Check sheet for the modelled part. Datum: model origin and axes. Units: mm. Face numbers are marked on the shaded views. A direction names the side the tool comes from. Give positions to 0.01 mm unless a question says otherwise; leave off trailing zeros. Write each loop counter-clockwise with the first axis right and the second up, starting at its lowest first coordinate (ties: lowest second). Pieces come first, ordered by that corner, then holes.
from build123d import *

# Parameters (mm, degrees)
SKETCH003_W          = 205
SKETCH003_H          = 151
PAD001_DEPTH         = 40
POCKET002_DEPTH      = 38
SKETCH005_R          = 15
POCKET003_DEPTH      = 2.001
POCKET003_DEPTH_BACK = 38.001
POCKET004_DEPTH      = 38


with BuildPart() as part:
    # Sketch003 → Pad001 (new body)
    with BuildSketch(Plane.XY):
        Rectangle(SKETCH003_W, SKETCH003_H)
    extrude(amount=PAD001_DEPTH)

    # Sketch004 (on Face6 of Pad001) → Pocket002 (cut)
    with BuildSketch(Plane.XY.offset(40)):
        Polygon((-101.5, 0), (-81.2, 35.160631), (-40.6, 35.160631), (-20.3, 70.321263), (20.3, 70.321263), (40.6, 35.160631), (81.2, 35.160631), (101.5, 0), (81.2, -35.160631), (40.6, -35.160631), (19.516262, -71.678737), (-19.516262, -71.678737), (-40.6, -35.160631), (-81.2, -35.160631), align=None)
    extrude(amount=-POCKET002_DEPTH, mode=Mode.SUBTRACT)

    # Sketch005 → Pocket003 (cut, two sides)
    with BuildSketch(Plane.XY.offset(2)) as pocket003_sk:
        with Locations((105, 0)):
            Circle(SKETCH005_R)
        with Locations((0, 75)):
            Circle(SKETCH005_R)
        with Locations((0, -75)):
            Circle(SKETCH005_R)
        with Locations((-105, 0)):
            Circle(SKETCH005_R)
    extrude(amount=-POCKET003_DEPTH, mode=Mode.SUBTRACT)
    extrude(pocket003_sk.sketch, amount=POCKET003_DEPTH_BACK, mode=Mode.SUBTRACT)

    # Sketch006 (on Face6 of Pad001) → Pocket004 (cut)
    with BuildSketch(Plane.XY.offset(40)):
        with BuildLine():
            ThreePointArc((-83.5, -39), (-100.5, -56), (-83.5, -73))
            Line((-83.5, -73), (-50, -73))
            ThreePointArc((-50, -73), (-33, -56), (-50, -39))
            Line((-50, -39), (-83.5, -39))
        make_face()
        with BuildLine():
            ThreePointArc((50, -39), (33, -56), (50, -73))
            Line((50, -73), (83.5, -73))
            ThreePointArc((83.5, -73), (100.5, -56), (83.5, -39))
            Line((83.5, -39), (50, -39))
        make_face()
        with BuildLine():
            ThreePointArc((50, 73), (33, 56), (50, 39))
            Line((50, 39), (83.5, 39))
            ThreePointArc((83.5, 39), (100.5, 56), (83.5, 73))
            Line((83.5, 73), (50, 73))
        make_face()
        with BuildLine():
            ThreePointArc((-83.5, 73), (-100.5, 56), (-83.5, 39))
            Line((-83.5, 39), (-50, 39))
            ThreePointArc((-50, 39), (-33, 56), (-50, 73))
            Line((-50, 73), (-83.5, 73))
        make_face()
    extrude(amount=-POCKET004_DEPTH, mode=Mode.SUBTRACT)


with BuildPart() as part_1:
    # Body001 placement: moved
    add(part.part.moved(Location((100, -60, 0))))


solid = part_1.part
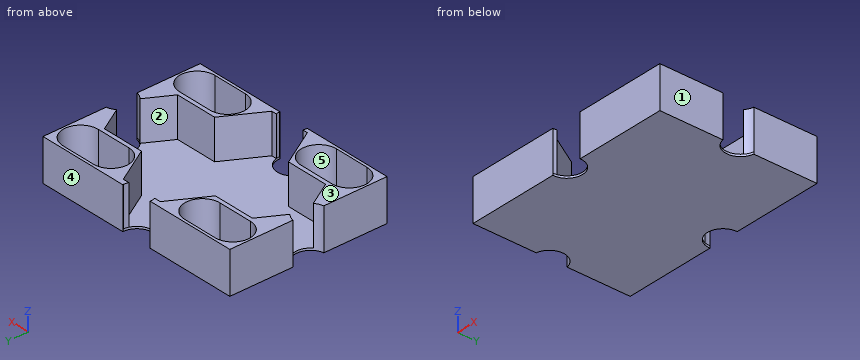
1) Sectioned sample at A-A on x = 43. Record the boundary of the cut face in (y, z).
2) Access from +Z, -Z, +X, -X, +Y, -Y to the whole of each face (thin tool, end or side, straight path). Record for the marked faces 1 and 2.
3) Sectioned sample at C-C on y = -91.5. Record the boundary of the cut face in (x, z), then the cut area to 3 significant figures.
4) Gauge pin test, flat ends, axial feed: pin 1 (17 mm diameter, centred on x = 155.5, y = -108.5, fed in from +Z); pin 2 (10 mm diameter, centred on x = 102.5, z = 5.5, fed in from +Y). Record the tip position at first contact, or that the pin passes through.
5) Scan lines: L1, parallel to Y at x = 50, z = 29; L2, parallel to X at y = -15.5, z = 31; L3, parallel to Y at x = 14, z = 20.5. Record each from-to range of solid material in increasing order.
6) Draft check along Y on the marked faces 3, 4 and 5. Enter one of: +Y half, -Y half, draft (parallel to the pull), parting line (faces both ways), or undercut.
7) Sectioned sample at D-D on y = -4. Record the boundary of the cut face in (x, z), then the cut area to 3 significant figures.
8) Sectioned sample at B-B on z = 19. Give the number of separate pieces and of enclosed holes in the cut face, then the cut area to 3 significant figures.
Answers below:
1. outline: (-135.5, 0) - (15.5, 0) - (15.5, 40) - (13, 40) - (13, 2) - (-21, 2) - (-21, 40) - (-24.84, 40) - (-24.84, 2) - (-95.16, 2) - (-95.16, 40) - (-99, 40) - (-99, 2) - (-133, 2) - (-133, 40) - (-135.5, 40) - close
2. face 1: +Z, -Z, +X, +Y, -Y
2. face 2: +Z
3. outline: (-2.5, 0) - (202.5, 0) - (202.5, 40) - (183.31, 40) - (183.31, 2) - (16.69, 2) - (16.69, 40) - (-2.5, 40) - close
3. area: 1,870 mm2
4. pin 1: stops at z = 2
4. pin 2: stops at y = 1.28
5. L1: y = -135.5 to -133, -99 to -95.16, -24.84 to -21, 13 to 15.5
5. L2: x = -2.5 to 3.98, 62.52 to 64.79, 135.21 to 137.48, 196.02 to 202.5
5. L3: y = -135.5 to -132.82, -99.18 to -86.85, -33.15 to -20.82, 12.82 to 15.5
6. face 3: draft
6. face 4: +Y half
6. face 5: undercut
7. outline: (-2.5, 0) - (202.5, 0) - (202.5, 40) - (200.5, 40) - (200.5, 2) - (133, 2) - (133, 40) - (128.57, 40) - (128.57, 2) - (71.43, 2) - (71.43, 40) - (67, 40) - (67, 2) - (-0.5, 2) - (-0.5, 40) - (-2.5, 40) - close
7. area: 899 mm2
8. separate pieces: 4
8. enclosed holes: 4
8. area: 5,060 mm2
